Source: CAD feature listing. Evaluate the final solid. Frame: model axes, mm. Face numbers are marked on the shaded views. A direction names the side the tool comes from. Give positions to 0.01 mm unless a question says otherwise; leave off trailing zeros. Order: outer loops, then holes, each group sorted by start corner. A loop starts at its lowest first (then second) coordinate and runs counter-clockwise, first axis right, second up.
1) Draft query along Y for the marked faces 1, 2, 3 and 4. Return one class per face: released by +Y, released by -Y, zero draft, split by the parting line, or undercut.
2) Material intervals for line 1 (Y direction, x = 0, z = 7); line 2 (Z direction, x = 15, y = -10); line 3 (Y direction, x = -2, z = 11), sorted ascending.
3) Section C-C, the plane z = -1.5. Give the number of separate pieces and of enclosed holes in the cut face, plus the area to 3 significant figures.
4) Section B-B, the plane y = 0. Return loops of the section in (x, z).
5) Access query for the marked faces 5 and 6. Directions: +Z, -Z, +X, -X, +Y, -Y. A direction counts if a zero-diameter tool reaches every point of the face in a straight line with its end or side. Return the directions, or none.
6) Section D-D, the plane z = 25. Return loops of the section in (x, y), plus the area to 3 significant figures.
7) Section A-A, the plane x = 0. Return loops of the section in (y, z).
8) First-contact query: P1, Ø5, axis at y = 13.5, z = 10.5, coming from the +X side; P2, Ø3, axis at y = 4.5, z = 13.5, coming from the +X side; P3, Ø20.5, axis at x = 45.05, y = 0, coming from the +Z side; P4, Ø11.5, axis at x = 0, y = 0, coming from the -Z side (3 decimals). Flat tips, straight axial feed; report the tip coordinate or a pass-through.
```python
from build123d import *
from build123d.topology import SkipClean

# Parameters (mm, degrees)
SKETCH1_R           = 6.35
SKETCH1_R_2         = 7.9375
BOSS_EXTRUDE1_DEPTH = 5.55625
BOSS_EXTRUDE2_START = 14.2875
SKETCH2_R           = 30.1625
SKETCH2_R_2         = 6.35
BOSS_EXTRUDE2_DEPTH = 14.2875
SKETCH3_R           = 11
SKETCH3_R_2         = 6.35
BOSS_EXTRUDE3_DEPTH = 7.9375


with BuildPart() as part:
    # Sketch1 → Boss-Extrude1 (new, symmetric)
    with BuildSketch(Plane.XY):
        with BuildLine():
            Line((-49.778964758, 10.272771945), (-12.623072687, 27.39405852))
            ThreePointArc((-12.623072687, 27.39405852), (0, 30.1625), (12.623072687, 27.39405852))
            Line((12.623072687, 27.39405852), (49.778964758, 10.272771945))
            ThreePointArc((49.778964758, 10.272771945), (56.35625, 0), (49.778964758, -10.272771945))
            Line((49.778964758, -10.272771945), (12.623072687, -27.39405852))
            ThreePointArc((12.623072687, -27.39405852), (0, -30.1625), (-12.623072687, -27.39405852))
            Line((-12.623072687, -27.39405852), (-49.778964758, -10.272771945))
            ThreePointArc((-49.778964758, -10.272771945), (-56.35625, 0), (-49.778964758, 10.272771945))
        make_face()
        Circle(SKETCH1_R, mode=Mode.SUBTRACT)
        with Locations((-45.0453125, 0)):
            Circle(SKETCH1_R_2, mode=Mode.SUBTRACT)
        with Locations((45.0453125, 0)):
            Circle(SKETCH1_R_2, mode=Mode.SUBTRACT)
    extrude(amount=BOSS_EXTRUDE1_DEPTH, both=True)

    # Sketch2 → Boss-Extrude2 (add)
    with SkipClean():  # the faces are left unmerged after this step: merging them gives an invalid solid
        with BuildSketch(Plane.XY.offset(5.55625).offset(BOSS_EXTRUDE2_START)):
            with Locations(Location((0, 0, 0), (0, 0, 114.740061343))):
                Circle(SKETCH2_R)
            Circle(SKETCH2_R_2, mode=Mode.SUBTRACT)
        extrude(amount=-BOSS_EXTRUDE2_DEPTH)

    # Sketch3 → Boss-Extrude3 (add)
    with SkipClean():  # the faces are left unmerged after this step: merging them gives an invalid solid
        with BuildSketch(Plane.XY.offset(19.84375)):
            Circle(SKETCH3_R)
            Circle(SKETCH3_R_2, mode=Mode.SUBTRACT)
        extrude(amount=BOSS_EXTRUDE3_DEPTH)


solid = part.part
```
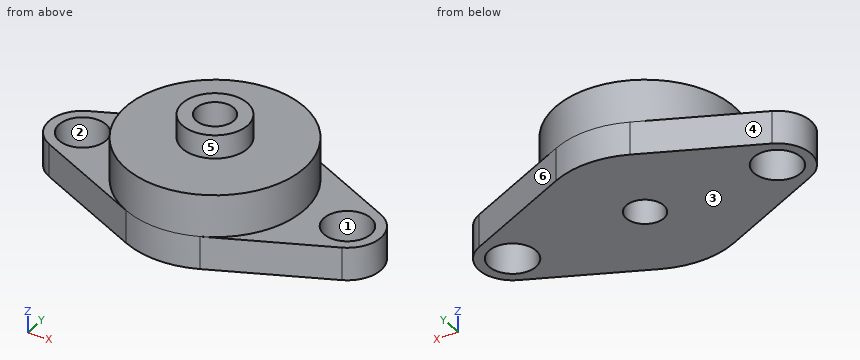
From the geometry:
1. face 1: undercut
1. face 2: undercut
1. face 3: zero draft
1. face 4: released by +Y
2. line 1: y = -30.16 to -6.35, 6.35 to 30.16
2. line 2: z = -5.56 to 19.84
2. line 3: y = -30.1 to -6.03, 6.03 to 30.1
3. separate pieces: 1
3. enclosed holes: 3
3. area: 3,950 mm2
4. outline: (-56.36, -5.56) - (-52.98, -5.56) - (-52.98, 5.56) - (-56.36, 5.56) - close; (-37.11, -5.56) - (-6.35, -5.56) - (-6.35, 27.78) - (-11, 27.78) - (-11, 19.84) - (-30.16, 19.84) - (-30.16, 5.56) - (-37.11, 5.56) - close; (6.35, -5.56) - (37.11, -5.56) - (37.11, 5.56) - (30.16, 5.56) - (30.16, 19.84) - (11, 19.84) - (11, 27.78) - (6.35, 27.78) - close; (52.98, -5.56) - (56.36, -5.56) - (56.36, 5.56) - (52.98, 5.56) - close
5. face 5: +Z
5. face 6: +Z, -Z, +X, +Y
6. outline: circle Ø22 at (0, 0); hole circle Ø12.7 at (0, 0)
6. area: 253 mm2
7. outline: (-30.16, -5.56) - (-6.35, -5.56) - (-6.35, 27.78) - (-11, 27.78) - (-11, 19.84) - (-30.16, 19.84) - close; (6.35, -5.56) - (30.16, -5.56) - (30.16, 19.84) - (11, 19.84) - (11, 27.78) - (6.35, 27.78) - close
8. P1: stops at x = 28.09
8. P2: stops at x = 30.01
8. P3: stops at z = 5.56
8. P4: passes through
